```python
from build123d import *

# Parameters (mm, degrees)
SKETCH1_W           = 70
SKETCH1_H           = 430
SKETCH1_W_2         = 50.4
SKETCH1_H_2         = 9.8
SKETCH1_W_3         = 49.8
SKETCH1_H_3         = 9.2
SKETCH1_W_4         = 49.9
SKETCH1_H_4         = 9.3
SKETCH1_W_5         = 50
SKETCH1_H_5         = 9.4
SKETCH1_W_6         = 50.1
SKETCH1_H_6         = 9.5
SKETCH1_W_7         = 50.2
SKETCH1_H_7         = 9.6
SKETCH1_W_8         = 50.3
SKETCH1_H_8         = 9.7
BOSS_EXTRUDE1_DEPTH = 10
M4_TAPPED_HOLE1_D   = 3.3


with BuildPart() as part:
    # Sketch1 → Boss-Extrude1 (new body)
    with BuildSketch(Plane.XY):
        Rectangle(SKETCH1_W, SKETCH1_H)
        with Locations((0, 166.8)):
            Rectangle(SKETCH1_W_2, SKETCH1_H_2, mode=Mode.SUBTRACT)
        with Locations((0, -170.4)):
            Rectangle(SKETCH1_W_3, SKETCH1_H_3, mode=Mode.SUBTRACT)
        with Locations((0, -114.45)):
            Rectangle(SKETCH1_W_4, SKETCH1_H_4, mode=Mode.SUBTRACT)
        with Locations((0, -58.4)):
            Rectangle(SKETCH1_W_5, SKETCH1_H_5, mode=Mode.SUBTRACT)
        with Locations((0, -2.25)):
            Rectangle(SKETCH1_W_6, SKETCH1_H_6, mode=Mode.SUBTRACT)
        with Locations((0, 54)):
            Rectangle(SKETCH1_W_7, SKETCH1_H_7, mode=Mode.SUBTRACT)
        with Locations((0, 110.35)):
            Rectangle(SKETCH1_W_8, SKETCH1_H_8, mode=Mode.SUBTRACT)
    extrude(amount=BOSS_EXTRUDE1_DEPTH)

    # M4 Tapped Hole1 (through all)
    with Locations(Plane.XY.offset(10)):
        with Locations((-25, -189.7), (25, -189.7), (25, -207), (-25, -207), (-25, -133.8), (25, -133.8), (25, -151.1), (-25, -151.1), (-25, -77.8), (25, -77.8), (25, -95.1), (-25, -95.1), (-25, -21.7), (25, -21.7), (25, -39), (-25, -39), (-25, 34.5), (25, 34.5), (25, 17.2), (-25, 17.2), (-25, 90.8), (25, 90.8), (25, 73.5), (-25, 73.5), (-25, 147.2), (25, 147.2), (25, 129.9), (-25, 129.9), (-25, 203.7), (25, 203.7), (25, 186.4), (-25, 186.4)):
            Hole(M4_TAPPED_HOLE1_D / 2)


solid = part.part
```
The listing builds one solid part. Answer for the finished solid, in the listing's coordinates (mm). A direction names the side the tool comes from. Give positions to 0.01 mm unless a question says otherwise; leave off trailing zeros. Write each question's results on one line, items separated by ' | '.
Q1. Section A-A, the plane x = 2 is taken. Count the separate pieces of the cut face and the enclosed holes in it, then the cut area to 4 significant figures.
Output values:
separate pieces: 8 | enclosed holes: 0 | area: 3,635 mm2
Q2. Consider L1, parallel to X at y = 203.7, z = 2.5; L2, parallel to X at y = -4, z = 5.75; L3, parallel to X at y = 92, z = 1.5. Determine where each line is inside the solid, lowest interval first. Write a range as from..to.
Output values:
L1: -35..-26.65, -23.35..23.35, 26.65..35 | L2: -35..-25.05, 25.05..35 | L3: -35..-26.13, -23.87..23.87, 26.13..35
Q3. A flat-ended cylindrical pin translates along its axis: P1, Ø2.5, axis at x = 25, y = -133.8, coming from the +Z side. Find the tip coordinate at first contact, or state that the pin passes through.
Output values:
P1: through
Q4. A tool of negligible diameter and unlimited length cuts with its end or side. For faces 1 (the flat face through (0, 49.2, 5)), 2 (the flat face through (35, -3, 5)), from which of +Z, -Z, +X, -X, +Y, -Y can it reach the whole face along a straight path? Write none if from no direction.
Output values:
face 1: +Z, -Z | face 2: +Z, -Z, +X, +Y, -Y
Q5. For a pull along Y with two mould halves and no side action, classify faces 3 (the flat face through (25.1, 54, 5)), 4 (the flat face through (0, 3, 0)), 5 (the flat face through (0, 215, 5)) as released by +Y, released by -Y, zero draft, split by the parting line, or undercut.
Output values:
face 3: undercut | face 4: zero draft | face 5: released by +Y
